Source: CAD feature listing. Evaluate the final solid. Frame: model axes, mm. Give positions to 0.01 mm unless a question says otherwise; leave off trailing zeros. Loops run counter-clockwise (first coordinate to the right, second up) from the corner with the lowest first, then second, coordinate; pieces in that order, holes last.
from build123d import *

# Parameters (mm, degrees)
EXTRUDE_1_DEPTH = 1.5


with BuildPart() as part:
    # 草图1 → 拉伸1 (new, symmetric)
    with BuildSketch(Plane(origin=(0, 0, 0), x_dir=(1, 0, 0), z_dir=(0, 1, 0))):
        with BuildLine():
            Line((20.940011064, 1.58846533), (20.939920521, 1.58736529))
            ThreePointArc((20.939920521, 1.58736529), (0.761777461, -20.986178668), (-20.999899431, 0.064991443))
            add(Edge.make_bspline(
                [(-8.051332909, 32.78715945), (-8.610349318, 32.182398754), (-9.714361715, 30.939196238), (-11.751951037, 28.441519755), (-14.028887881, 25.244274154), (-16.311662528, 21.307878415), (-18.150397892, 17.266249907), (-19.545128941, 13.120876546), (-20.496807064, 8.86508597), (-21.004475075, 4.530924038), (-21.049002229, 1.538986899), (-20.999899431, 0.064991443)],
                knots=[0.004872267, 0.004872267, 0.004872267, 0.004872267, 0.02895963, 0.053109791, 0.101410114, 0.149710437, 0.198010759, 0.246311082, 0.294611405, 0.342911728, 0.39069527, 0.39069527, 0.39069527, 0.39069527], degree=3))
            Line((-8.051332909, 32.78715945), (-8.072524116, 33.5))
            add(Edge.make_bspline(
                [(-8.072524116, 33.5), (-22.136696557, 18.527333844), (-21.5, 0)],
                knots=[0, 0, 0, 0.391212051, 0.391212051, 0.391212051], degree=2))
            ThreePointArc((-21.5, 0), (0.807061405, -21.48484703), (21.439409478, 1.612985193))
            add(Edge.make_bspline(
                [(10.927475884, 34.265791626), (20.575756572, 19.203087379), (21.439409478, 1.612985193)],
                knots=[0, 0, 0, 0.204404978, 0.204404978, 0.204404978], degree=2))
            Line((10.927475884, 34.265791626), (10.588152757, 34.734289031))
            Line((10.588152757, 34.734289031), (10.236755206, 34.417135424))
            add(Edge.make_bspline(
                [(10.236755206, 34.417135424), (11.041253847, 33.161168119), (12.610265397, 30.600103215), (15.317060933, 25.402889951), (18.018451366, 18.698039733), (19.779296418, 11.724493606), (20.629070045, 5.992876218), (20.868076786, 3.053557708), (20.940011064, 1.58846533)],
                knots=[-0.002856761, -0.002856761, -0.002856761, -0.002856761, 0.023050957, 0.048958674, 0.100774109, 0.152589544, 0.178497261, 0.204404978, 0.204404978, 0.204404978, 0.204404978], degree=3))
        make_face()
    extrude(amount=EXTRUDE_1_DEPTH, both=True)


solid = part.part
1) Ray query, probe 1 along X at (y, z) = (0.8, -6.5); probe 2 along X at (y, z) = (1.35, 8); probe 3 along Z at (x, y) = (-12, 0.95). Return the intervals inside material, ascending.
Checks:
probe 1: x = -21.26 to -20.75, 20.52 to 21.02
probe 2: x = -19.96 to -19.42, 19.42 to 19.96
probe 3: z = -28.88 to -28.04, 17.23 to 17.84
2) Cut plane C-C (x = 6.5). Return loops of the section in (y, z).
Checks:
outline: (-1.5, 19.97) - (1.5, 19.97) - (1.5, 20.49) - (-1.5, 20.49) - close
3) Cut plane B-B (x = 0). Return loops of the section in (y, z).
Checks:
outline: (-1.5, 21) - (1.5, 21) - (1.5, 21.5) - (-1.5, 21.5) - close
4) Pull-direction query (X, two-part tool) for faces 1 (the flat face through (16, 1.5, 14)), 2 (the cylindrical face through (0.323, 0.021, 21.498)), 3 (the cylindrical face through (1.235, 0.021, 20.964)); classes: released by +X, released by -X, zero draft, split by the parting line, or undercut.
Checks:
face 1: zero draft
face 2: split by the parting line
face 3: undercut
5) Cut plane A-A (z = 14). Return loops of the section in (x, y), and give its area (3 significant figures).
Checks:
outline: (-16.32, -1.5) - (-15.65, -1.5) - (-15.65, 1.5) - (-16.32, 1.5) - close; (15.65, -1.5) - (16.32, -1.5) - (16.32, 1.5) - (15.65, 1.5) - close
area: 3.99 mm2
6) Contact query for flat-ended pins moving along their axis: P1, Ø1.5, axis at x = 4.5, y = -0.5, coming from the -Z side; P2, Ø1.5, axis at x = -14, y = -0.5, coming from the -Z side; P3, Ø12, axis at x = -10, z = -13.5, coming from the +Y side; P4, Ø1.5, axis at x = -2.5, y = 1, coming from the -Z side. Output: stop coordinate, or through.
Checks:
P1: stops at z = 20.33
P2: stops at z = -27.17
P3: passes through
P4: stops at z = 20.75
